Verification items for the finished model (mm, model axes). Face numbers are marked on the shaded views. A direction names the side the tool comes from. Round coordinates to 2 decimals unless told otherwise and drop trailing zeros. Write each loop counter-clockwise with the first axis right and the second up, starting at its lowest first coordinate (ties: lowest second). Pieces come first, ordered by that corner, then holes. Notation, with made-up numbers: (-17.5, 35) - (9.5, 35) arc R8 cw to (9.5, 49) - close; hole circle Ø5 at (89.25, 34.25). An arc over 180 degrees is marked (long way). Answer as a JSON object with one key per item and string values.
```python
from build123d import *

# Parameters (mm, degrees)
FLANGE_BASE1_DEPTH    = 12.7
ESBO_O3_R             = 5
CORTE_EXTRUS_O1_DEPTH = 10


# Sheet-metal steps are written as plain solids
with BuildPart() as part:
    # Esboço1 → Flange-base1 (new, symmetric)
    with BuildSketch(Plane.XY):
        with BuildLine():
            Line((-65, 0), (-29.35, 0))
            ThreePointArc((-29.35, 0), (-26.274085502, 1.274085502), (-25, 4.35))
            Line((-25, 4.35), (-25, 49))
            ThreePointArc((-25, 49), (-24.707106781, 49.707106781), (-24, 50))
            Line((-24, 50), (24, 50))
            ThreePointArc((24, 50), (24.707106781, 49.707106781), (25, 49))
            Line((25, 49), (25, 4.35))
            ThreePointArc((25, 4.35), (26.274085502, 1.274085502), (29.35, 0))
            Line((29.35, 0), (65, 0))
            Line((65, 0), (65, 3.35))
            Line((65, 3.35), (29.35, 3.35))
            ThreePointArc((29.35, 3.35), (28.642893219, 3.642893219), (28.35, 4.35))
            Line((28.35, 4.35), (28.35, 49))
            ThreePointArc((28.35, 49), (27.075914498, 52.075914498), (24, 53.35))
            Line((24, 53.35), (-24, 53.35))
            ThreePointArc((-24, 53.35), (-27.075914498, 52.075914498), (-28.35, 49))
            Line((-28.35, 49), (-28.35, 4.35))
            ThreePointArc((-28.35, 4.35), (-28.642893219, 3.642893219), (-29.35, 3.35))
            Line((-29.35, 3.35), (-65, 3.35))
            Line((-65, 3.35), (-65, 0))
        make_face()
    extrude(amount=FLANGE_BASE1_DEPTH, both=True)

    # Esboço3 → Corte-extrusão1 (cut)
    with BuildSketch(Plane.XZ):
        with Locations((47, 0)):
            Circle(ESBO_O3_R)
        with Locations(Location((-47, 0, 0), (0, 0, 180))):
            Circle(ESBO_O3_R)
    extrude(amount=-CORTE_EXTRUS_O1_DEPTH, mode=Mode.SUBTRACT)


solid = part.part
```
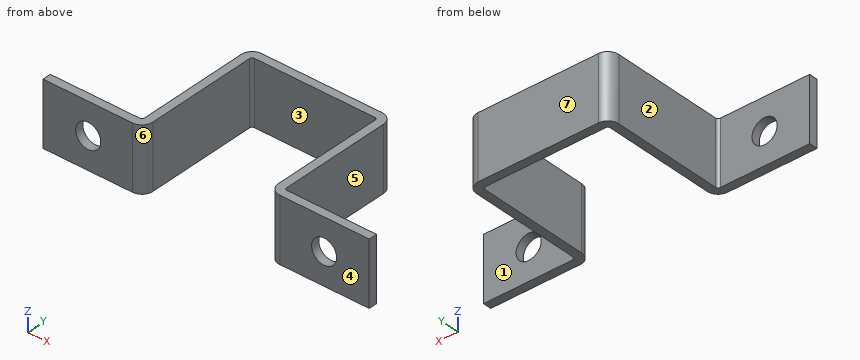
1. Access from +Z, -Z, +X, -X, +Y, -Y to the whole of each face (thin tool, end or side, straight path). Record for the marked faces 1, 2, 3 and 4.
Completed:
{"face 1": "+Z, -Z, +X, +Y", "face 2": "+Z, -Z, -X, +Y", "face 3": "+Z, -Z, -Y", "face 4": "+Z, -Z, +X, -X, -Y"}
2. Cross-section at D-D (z = 6.5). Record the boundary of the cut face in (x, y), plus the area to 3 significant figures.
Completed:
{"outline": "(-65, 0) - (-29.35, 0) arc R4.35 ccw to (-25, 4.35) - (-25, 49) arc R1 cw to (-24, 50) - (24, 50) arc R1 cw to (25, 49) - (25, 4.35) arc R4.35 ccw to (29.35, 0) - (65, 0) - (65, 3.35) - (29.35, 3.35) arc R1 cw to (28.35, 4.35) - (28.35, 49) arc R4.35 ccw to (24, 53.35) - (-24, 53.35) arc R4.35 ccw to (-28.35, 49) - (-28.35, 4.35) arc R1 cw to (-29.35, 3.35) - (-65, 3.35) - close", "area": "755 mm^2"}
3. Cross-section at A-A (x = 47). Record the boundary of the cut face in (y, z).
Completed:
{"outline": "(0, -12.7) - (3.35, -12.7) - (3.35, -5) - (0, -5) - close; (0, 5) - (3.35, 5) - (3.35, 12.7) - (0, 12.7) - close"}
4. Material ranges on probe 1 along Z at (x, y) = (-47, 2); probe 2 along X at (y, z) = (35.5, 8.75); probe 3 along X at (y, z) = (2.5, 2), recorded low to high. Write a range as from..to.
Completed:
{"probe 1": "z = -12.7..-5, 5..12.7", "probe 2": "x = -28.35..-25, 25..28.35", "probe 3": "x = -65..-51.58, -42.42..-25.41, 25.41..42.42, 51.58..65"}
5. Mould release check, pull along X, two halves, no side actions. Record for the marked faces 5, 6 and 7: released by +X, released by -X, zero draft, split by the parting line, or undercut.
Completed:
{"face 5": "released by +X", "face 6": "undercut", "face 7": "zero draft"}
6. Cross-section at C-C (y = 34.5). Record the boundary of the cut face in (x, z), plus the area to 3 significant figures.
Completed:
{"outline": "(-28.35, -12.7) - (-25, -12.7) - (-25, 12.7) - (-28.35, 12.7) - close; (25, -12.7) - (28.35, -12.7) - (28.35, 12.7) - (25, 12.7) - close", "area": "170 mm^2"}
7. Cross-section at B-B (z = -3). Record the boundary of the cut face in (x, y).
Completed:
{"outline": "(-65, 0) - (-51, 0) - (-51, 3.35) - (-65, 3.35) - close; (-43, 0) - (-29.35, 0) arc R4.35 ccw to (-25, 4.35) - (-25, 49) arc R1 cw to (-24, 50) - (24, 50) arc R1 cw to (25, 49) - (25, 4.35) arc R4.35 ccw to (29.35, 0) - (43, 0) - (43, 3.35) - (29.35, 3.35) arc R1 cw to (28.35, 4.35) - (28.35, 49) arc R4.35 ccw to (24, 53.35) - (-24, 53.35) arc R4.35 ccw to (-28.35, 49) - (-28.35, 4.35) arc R1 cw to (-29.35, 3.35) - (-43, 3.35) - close; (51, 0) - (65, 0) - (65, 3.35) - (51, 3.35) - close"}
8. Go/stop test with flat-tipped pins: pin 1 (10 mm diameter, centred on y = 27, z = -6.5, fed in from -X); pin 2 (8 mm diameter, centred on y = 34.5, z = 1.5, fed in from +X); pin 3 (10 mm diameter, centred on x = -16, y = 10.5, fed in from -Z); pin 4 (8 mm diameter, centred on x = -48, z = 5, fed in from +Y). Record where each tip stops, or that it passes through.
Completed:
{"pin 1": "stops at x = -28.35", "pin 2": "stops at x = 28.35", "pin 3": "passes through", "pin 4": "stops at y = 3.35"}
